from build123d import *

# Parameters (mm, degrees)
DIAM_TRE_DU_PER_AGE_1_0_1_1_D     = 1
DIAM_TRE_DU_PER_AGE_1_0_1_1_DEPTH = 2
DIAM_TRE_DU_PER_AGE_1_0_1_1_TIP   = 0.30043031
DIAM_TRE_DU_PER_AGE_5_0_5_1_D     = 5
DIAM_TRE_DU_PER_AGE_5_0_5_1_DEPTH = 9.5
DIAM_TRE_DU_PER_AGE_5_0_5_1_TIP   = 1.502151548


with BuildPart() as part:
    # Esquisse7 → Révolution2 (revolve)
    with BuildSketch(Plane.XY, mode=Mode.PRIVATE) as r_volution2_sk:
        Polygon((0, 15), (0, 18), (-19, 18), (-19, 15), (-20, 15), (-20, 16), (-23, 16), (-24, 15), (-24, 8), (-23, 8), (-23, 0), (-10.5, 0), (-10.5, 4.75), (-11.25, 5.5), (-19.75, 5.5), (-20.5, 6.25), (-20.5, 11.75), (-19.75, 12.5), (-15.5, 12.5), (-13, 15), (-8, 15), (-8, 16), (-7, 16), (-7, 15), align=None)
    revolve(r_volution2_sk.sketch.rotate(Axis((-24, 0, 0), (1, 0, 0)), 90), axis=Axis((-24, 0, 0), (1, 0, 0)))

    # Diamètre du perçage Ø1.0 (1)1
    with Locations(Plane(origin=(-10.5, 0, 0), x_dir=(0, 0, -1), z_dir=(1, 0, 0))):
        with Locations((0, 0)):
            Hole(DIAM_TRE_DU_PER_AGE_1_0_1_1_D / 2, depth=DIAM_TRE_DU_PER_AGE_1_0_1_1_DEPTH)
            with Locations((0, 0, -(DIAM_TRE_DU_PER_AGE_1_0_1_1_DEPTH + DIAM_TRE_DU_PER_AGE_1_0_1_1_TIP / 2))):  # 118° drill point
                Cone(0, DIAM_TRE_DU_PER_AGE_1_0_1_1_D / 2, DIAM_TRE_DU_PER_AGE_1_0_1_1_TIP, mode=Mode.SUBTRACT)

    # Diamètre du perçage Ø5.0 (5)1
    with Locations(Plane.ZY.offset(23)):
        with Locations((0, 0)):
            Hole(DIAM_TRE_DU_PER_AGE_5_0_5_1_D / 2, depth=DIAM_TRE_DU_PER_AGE_5_0_5_1_DEPTH)
            with Locations((0, 0, -(DIAM_TRE_DU_PER_AGE_5_0_5_1_DEPTH + DIAM_TRE_DU_PER_AGE_5_0_5_1_TIP / 2))):  # 118° drill point
                Cone(0, DIAM_TRE_DU_PER_AGE_5_0_5_1_D / 2, DIAM_TRE_DU_PER_AGE_5_0_5_1_TIP, mode=Mode.SUBTRACT)


solid = part.part
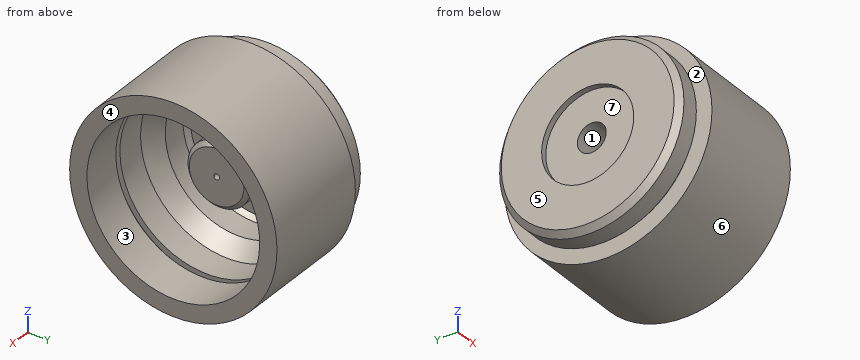
Read the model definition and answer for the solid it produces. Units are mm, in the model's axes. Face numbers are marked on the shaded views. A direction names the side the tool comes from. Round coordinates to 2 decimals unless told otherwise and drop trailing zeros. Write each loop counter-clockwise with the first axis right and the second up, starting at its lowest first coordinate (ties: lowest second). Pieces come first, ordered by that corner, then holes. Notation, with made-up numbers: (35.5, 25.5) - (93.5, 25.5) arc R21 cw to (93.5, 54.5) - close; hole circle Ø8 at (64.5, 0). An arc over 180 degrees is marked (long way). Use a Markdown table: item, result.
(1) The part is cut by section B-B (x = -1.75). Write down the section's boundary in (y, z), then the cut area to 3 significant figures.
Reported:
| item | result |
|---|---|
| outline | circle Ø36 at (0, 0); hole circle Ø30 at (0, 0) |
| area | 311 mm2 |
(2) Each of these flat-tipped pins is pushed along its axis until it touches: pin 1 Ø1 at (x, z) = (-21, -5) entering from -Y; pin 2 Ø19 at (y, z) = (0, 0) entering from +X; pin 3 Ø4 at (y, z) = (0, 0) entering from -X. Where does it stop, or does it pass through?
Reported:
| item | result |
|---|---|
| pin 1 | y = -15.35 |
| pin 2 | x = -10.5 |
| pin 3 | x = -13.2 |
(3) The part is cut by section A-A (x = -17.25). Write down the section's boundary in (y, z).
Reported:
| item | result |
|---|---|
| outline | circle Ø36 at (0, 0); circle Ø11 at (0, 0); hole circle Ø25 at (0, 0); hole circle Ø5 at (0, 0) |
(4) The mould has two halves that part along Z. Classify the marked faces 5, 6 and 7: released by +Z, released by -Z, zero draft, split by the parting line, or undercut.
Reported:
| item | result |
|---|---|
| face 5 | zero draft |
| face 6 | split by the parting line |
| face 7 | undercut |
(5) The part is cut by section C-C (x = -22.5). Write down the section's boundary in (y, z).
Reported:
| item | result |
|---|---|
| outline | circle Ø32 at (0, 0); hole circle Ø5 at (0, 0) |
(6) Straight lines are drawn through the part: line 1 along Y through (x, z) = (-17.85, 0); line 2 along Y through (x, z) = (-1.5, 0.5); line 3 along Y through (x, z) = (-7.45, 0). For each, find the intervals that lie inside material, in ascending order. Write a range as [from, to].
Reported:
| item | result |
|---|---|
| line 1 | [-18, -12.5], [-5.5, -2.5], [2.5, 5.5], [12.5, 18] |
| line 2 | [-17.99, -14.99], [14.99, 17.99] |
| line 3 | [-18, -16], [16, 18] |
(7) Which of the six approach directions +Z, -Z, +X, -X, +Y, -Y give full straight-line access (tool end or side, diameter ignored) to the marked faces 1, 2, 3 and 4?
Reported:
| item | result |
|---|---|
| face 1 | -X |
| face 2 | none |
| face 3 | +X |
| face 4 | +Z, -Z, +X, +Y, -Y |
